```python
from build123d import *

# Parameters (mm, degrees)
SKETCH_1_R               = 60
EXTRUDE_1_DEPTH          = 17
SKETCH_2_R               = 3.8
CUT_EXTRUDE_1_DEPTH      = 87.539008545
EXTRUDE_2_DEPTH          = 6.4
SKETCH_4_R               = 3
CUT_EXTRUDE_7_DEPTH      = 101.866049789
CUT_EXTRUDE_3_REACH      = 98.773
SKETCH_5_R               = 5
SKETCH_6_R               = 11.5
CUT_EXTRUDE_4_DEPTH      = 6
CUT_EXTRUDE_5_REACH      = 97.901
SKETCH_7_R               = 1.75
CUT_EXTRUDE_6_REACH      = 98.773
PATTERN_CIRCULAR_3_COUNT = 4
PATTERN_CIRCULAR_4_COUNT = 4


with BuildPart() as part:
    # Sketch 1 → Extrude 1 (new body)
    with BuildSketch(Plane.XY):
        Circle(SKETCH_1_R)
    extrude(amount=EXTRUDE_1_DEPTH)

    # Sketch 2 → Cut-Extrude 1 (cut, through all)
    with BuildSketch(Plane.XY.offset(17)):
        with Locations((-30, 30)):
            Circle(SKETCH_2_R)
        with Locations((30, 30)):
            Circle(SKETCH_2_R)
        with Locations((30, -30)):
            Circle(SKETCH_2_R)
        with Locations((-30, -30)):
            Circle(SKETCH_2_R)
    extrude(amount=-CUT_EXTRUDE_1_DEPTH, mode=Mode.SUBTRACT)

    # Sketch 3 → Extrude 2 (add, symmetric)
    with BuildSketch(Plane(origin=(0, 0, 0), x_dir=(0, 0, -1), z_dir=(1, 0, 0))):
        with BuildLine():
            Line((0, 58), (-16, 58))
            Line((-16, 58), (-16, 66))
            ThreePointArc((-16, 66), (-8, 74), (0, 66))
            Line((0, 66), (0, 58))
        make_face()
    extrude_2 = extrude(amount=EXTRUDE_2_DEPTH, both=True)

    # Sketch 4 → Cut-Extrude 7 (cut, through all)
    with BuildSketch(Plane(origin=(6.4, 0, 0), x_dir=(0, 0, -1), z_dir=(1, 0, 0))):
        with Locations((-8, 67.6576902)):
            Circle(SKETCH_4_R)
    cut_extrude_7 = extrude(amount=-CUT_EXTRUDE_7_DEPTH, mode=Mode.SUBTRACT)

    # Sketch 5 → Cut-Extrude 3 (cut, up to next)
    with BuildSketch(Plane(origin=(0, 0, 0), x_dir=(-1, 0, 0), z_dir=(0, 0, -1)), mode=Mode.PRIVATE) as cut_extrude_3_sk1:
        Circle(SKETCH_5_R)
    cut_extrude_3_tool1 = extrude(cut_extrude_3_sk1.sketch, amount=-CUT_EXTRUDE_3_REACH, mode=Mode.PRIVATE) & part.part
    add(cut_extrude_3_tool1.solids().sort_by_distance((0, 0, 0))[0], mode=Mode.SUBTRACT)

    # Sketch 6 → Cut-Extrude 4 (cut)
    with BuildSketch(Plane.XY.offset(17)):
        Circle(SKETCH_6_R)
    extrude(amount=-CUT_EXTRUDE_4_DEPTH, mode=Mode.SUBTRACT)

    # Sketch 7 → Cut-Extrude 5 (cut, up to next)
    with BuildSketch(Plane.XY.offset(11), mode=Mode.PRIVATE) as cut_extrude_5_sk1:
        with Locations((-8, 0)):
            Circle(SKETCH_7_R)
    cut_extrude_5_tool1 = extrude(cut_extrude_5_sk1.sketch, amount=-CUT_EXTRUDE_5_REACH, mode=Mode.PRIVATE) & part.part
    # Sketch 7 → Cut-Extrude 5 (cut, up to next)
    with BuildSketch(Plane.XY.offset(11), mode=Mode.PRIVATE) as cut_extrude_5_sk2:
        with Locations((0, 8)):
            Circle(SKETCH_7_R)
    cut_extrude_5_tool2 = extrude(cut_extrude_5_sk2.sketch, amount=-CUT_EXTRUDE_5_REACH, mode=Mode.PRIVATE) & part.part
    # Sketch 7 → Cut-Extrude 5 (cut, up to next)
    with BuildSketch(Plane.XY.offset(11), mode=Mode.PRIVATE) as cut_extrude_5_sk3:
        with Locations((8, 0)):
            Circle(SKETCH_7_R)
    cut_extrude_5_tool3 = extrude(cut_extrude_5_sk3.sketch, amount=-CUT_EXTRUDE_5_REACH, mode=Mode.PRIVATE) & part.part
    # Sketch 7 → Cut-Extrude 5 (cut, up to next)
    with BuildSketch(Plane.XY.offset(11), mode=Mode.PRIVATE) as cut_extrude_5_sk4:
        with Locations((0, -8)):
            Circle(SKETCH_7_R)
    cut_extrude_5_tool4 = extrude(cut_extrude_5_sk4.sketch, amount=-CUT_EXTRUDE_5_REACH, mode=Mode.PRIVATE) & part.part
    add(cut_extrude_5_tool1.solids().sort_by_distance((-8, 0, 11))[0], mode=Mode.SUBTRACT)
    add(cut_extrude_5_tool2.solids().sort_by_distance((0, 8, 11))[0], mode=Mode.SUBTRACT)
    add(cut_extrude_5_tool3.solids().sort_by_distance((8, 0, 11))[0], mode=Mode.SUBTRACT)
    add(cut_extrude_5_tool4.solids().sort_by_distance((0, -8, 11))[0], mode=Mode.SUBTRACT)

    # Sketch 8 → Cut-Extrude 6 (cut, up to next)
    with BuildSketch(Plane.XY.offset(17), mode=Mode.PRIVATE) as cut_extrude_6_sk1:
        with BuildLine():
            Line((-18.09189724, 12.423764363), (-31.926877482, 21.924290052))
            ThreePointArc((-31.926877482, 21.924290052), (-40.638216775, 23.204165271), (-46.984631039, 17.101007166))
            ThreePointArc((-46.984631039, 17.101007166), (-50, 0), (-46.984631039, -17.101007166))
            ThreePointArc((-46.984631039, -17.101007166), (-40.638216775, -23.204165271), (-31.926877482, -21.924290052))
            Line((-31.926877482, -21.924290052), (-18.09189724, -12.423764363))
            ThreePointArc((-18.09189724, -12.423764363), (-15.903129, -9.481080017), (-15.974774553, -5.814342437))
            ThreePointArc((-15.974774553, -5.814342437), (-17, 0), (-15.974774553, 5.814342437))
            ThreePointArc((-15.974774553, 5.814342437), (-15.903129, 9.481080017), (-18.09189724, 12.423764363))
        make_face()
    cut_extrude_6_tool1 = extrude(cut_extrude_6_sk1.sketch, amount=-CUT_EXTRUDE_6_REACH, mode=Mode.PRIVATE) & part.part
    cut_extrude_6 = cut_extrude_6_tool1.solids().sort_by_distance((-33.87223, 0, 17))[0]
    add(cut_extrude_6, mode=Mode.SUBTRACT)

    # Pattern Circular 3: Cut-Extrude 6 ×4 about axis
    pattern_circular_3_axis = Axis((0, 0, 0), (0, 0, 1))
    for i in range(1, PATTERN_CIRCULAR_3_COUNT):
        add(cut_extrude_6.rotate(pattern_circular_3_axis, i * 360 / PATTERN_CIRCULAR_3_COUNT), mode=Mode.SUBTRACT)

    # Pattern Circular 4: Extrude 2, Cut-Extrude 7 ×4 about axis
    pattern_circular_4_axis = Axis((0, 0, 0), (0, 0, 1))
    add([extrude_2.rotate(pattern_circular_4_axis, i * 360 / PATTERN_CIRCULAR_4_COUNT) for i in range(1, PATTERN_CIRCULAR_4_COUNT)])
    add([cut_extrude_7.rotate(pattern_circular_4_axis, i * 360 / PATTERN_CIRCULAR_4_COUNT) for i in range(1, PATTERN_CIRCULAR_4_COUNT)], mode=Mode.SUBTRACT)


solid = part.part
```
Can you work these out from the model? Positions are in its coordinate system, mm. A direction names the side the tool comes from. Round coordinates to 2 decimals unless told otherwise and drop trailing zeros. Loops run counter-clockwise (first coordinate to the right, second up) from the corner with the lowest first, then second, coordinate; pieces in that order, holes last. Notation, with made-up numbers: M 10.5,-9 L 45.5,-9 A15 cw 45.5,-5 Z; hole C -31.5,82.5 d6. An arc over 180 degrees is marked long. Answer as a JSON object with one key per item and string values. Group by question number.
Q1. Imagine slicing it at B-B, the plane y = 30. Please give me the cut outline in (x, z), then the cut area to 3 significant figures.
Q2. Will these pins go through, and if not, where does the flat tip stop? pin 1 (5 mm diameter, centred on y = 5.5, z = 1.5, fed in from -X); pin 2 (2 mm diameter, centred on x = -8, y = 0, fed in from +Z); pin 3 (8 mm diameter, centred on y = 67.66, z = 8, fed in from +X); pin 4 (7 mm diameter, centred on x = 67.66, z = 8, fed in from +Y).
Q3. Imagine slicing it at C-C, the plane z = 8. Count the separate pieces of the cut face and the enclosed holes in it, then the cut area to 3 significant figures.
Q4. Please list where these lines run through material, in increasing order: L1, parallel to Y at x = -20.5, z = 5; L2, parallel to Y at x = 12.5, z = 13; L3, parallel to Y at x = -13.5, z = 13.75.
Q5. We'd pull the mould along X, two halves only. Please class faces 4 (the flat face through (-64, 6.4, 8)), 5 (the cylindrical face through (-32.8, 32.57, 8.62)): +X half, -X half, draft (parallel to the pull), parting line (faces both ways), or undercut.
Q6. On a 3-axis mill with a long thin cutter (end or side, diameter ignored), from which of +Z, -Z, +X, -X, +Y, -Y can I reach the whole of each face in a straight line? I mean faces 1 (the cylindrical face through (0, 74, 8)), 2 (the flat face through (64, 6.4, 8)), 3 (the cylindrical face through (-50, 0, 9)). Say none if no direction works.
Q7. Imagine slicing it at A-A, the plane x = -44.5. Please give me the cut outline in (y, z), then the cut area to 3 significant figures.
Findings:
{
 "1": {"outline": "M -51.96,0 L -33.8,0 L -33.8,17 L -51.96,17 Z; M -26.2,0 L -20.6,0 L -20.6,17 L -26.2,17 Z; M 20.6,0 L 26.2,0 L 26.2,17 L 20.6,17 Z; M 33.8,0 L 51.96,0 L 51.96,17 L 33.8,17 Z", "area": "808 mm2"},
 "2": {"pin 1": "stops at x = -72.93", "pin 2": "passes through", "pin 3": "stops at x = 6.4", "pin 4": "stops at y = 6.4"},
 "3": {"separate pieces": "5", "enclosed holes": "13", "area": "6,390 mm2"},
 "4": {"L1": "y = -56.39 to -44.9, -29.85 to -14.08, 14.08 to 29.85, 44.9 to 56.39", "L2": "y = -58.68 to -48.41, -18.2 to 18.2, 48.41 to 58.68", "L3": "y = -58.46 to -48.14, -19.66 to 19.66, 48.14 to 58.46"},
 "5": {"face 4": "draft", "face 5": "undercut"},
 "6": {"face 1": "+X, -X, +Y", "face 2": "+Z, -Z, +X, +Y", "face 3": "+Z, -Z"},
 "7": {"outline": "M -40.25,0 L -20.91,0 L -20.91,17 L -40.25,17 Z; M 20.91,0 L 40.25,0 L 40.25,17 L 20.91,17 Z", "area": "658 mm2"}
}
